Autodesk Inventor part; units mm, degrees
ref_plane "Work Plane1" through (-10, 0, -166.5) normal (-1, 0, 0) x (0, -1, 0)
ref_plane "YZ Plane" through (0, 0, 0) normal (1, 0, 0) x (0, 1, 0)
ref_plane "XZ Plane" through (0, 0, 0) normal (0, 1, 0) x (-1, 0, 0)
sketch "Sketch1" plane through (0, 0, 0) normal (1, 0, 0) x (0, 1, 0)
  line L0 (0, 0) -> (5, 0)
  line L1 (5, 0) -> (5, -15)
  line L2 (5, -15) -> (10, -15)
  line L3 (10, -15) -> (10, -72)
  line L4 (10, -72) -> (15, -72)
  line L5 (15, -72) -> (15, -121.5)
  line L6 (15, -121.5) -> (10, -121.5)
  line L7 (10, -121.5) -> (10, -166.5)
  line L8 (10, -166.5) -> (0, -166.5)
  line L9 (0, -166.5) -> (0, -166.5)
  line L10 (0, -166.5) -> (0, -166.5)
  line L11 (0, -166.5) -> (0, 0)
  point P0 (0, -83.25)
  point P1 (15, -96.75)
  point P2 (5, -166.5)
  point P3 (2.5, 0)
  point P4 (12.5, -72)
  dimension "d0" = 15
  dimension "d1" = 5
  dimension "d3" = 10
  dimension "d4" = 49.5
  dimension "d5" = 15
  dimension "d6" = 45
  dimension "d7" = 0
  dimension "d8" = 0
  dimension "d9" = 72
revolve "Revolution1" add sketch "Sketch1" angle 360 about axis through (0, 0, -166.5) along (0, 0, 1)
sketch "Sketch2" plane through (0, 0, 0) normal (0, 0, 1) x (1, 0, 0)
  circle A0 centre (0, 0) radius 5
hole "Hole1" at (0, 0, 0) direction (0, 0, -1) diameter 5.9175 depth 19.1 tip angle 118
sketch "Sketch3" plane through (0, 0, -166.5) normal (0, 0, -1) x (-1, 0, 0)
  circle A0 centre (0, 0) radius 10
  line L0 (0, 0) -> (10, 0)
  circle A1 centre (0, 0) radius 10
ref_plane "Work Plane1" through (-10, 0, -166.5) normal (-1, 0, 0) x (0, -1, 0)
sketch "Sketch4" plane through (-10, 0, -166.5) normal (-1, 0, 0) x (0, -1, 0)
  line L0 (10, 45) -> (-10, 45)
  line L1 (10, 0) -> (-10, 0)
  line L2 (10, 0) -> (-10, 0)
  line L3 (0, 0) -> (-5.5, 0)
  line L4 (-5.5, 0) -> (-5.5, 13)
  line L5 (-5.5, 13) -> (5.5, 13) construction
  line L6 (5.5, 13) -> (5.5, 0)
  line L7 (0, 0) -> (5.5, 0)
  arc A0 (5.5, 13) -> (-5.5, 13) centre (0, 13) ccw
  point P0 (0, 166.5)
  point P1 (-5.5, 0)
  dimension "d18" = 5.5
  dimension "d19" = 13
  dimension "d20" = 11
extrude "Extrusion1" cut sketch "Sketch4" against normal blind 3
sketch "Sketch5" plane through (-7, -5.5, -166.5) normal (0, 0, -1) x (-1, 0, 0)
  point P0 (-7, 5.5)
  point P1 (-7, 5.5)
hole "Hole2" at (0, 0, -166.5) direction (0, 0, 1) diameter 5.9175 depth 19.1 tip angle 118
properties part number "SP002" material "Steel, Mild"
The listing builds one solid part. Answer for the finished solid, in the listing's coordinates (mm). A direction names the side the tool comes from. Coordinates: 2 decimals unless noted, no trailing zeros. Loops run counter-clockwise (first coordinate to the right, second up) from the corner with the lowest first, then second, coordinate; pieces in that order, holes last. Notation, with made-up numbers: (61.25, 29.5) -> (106.25, 29.5) arc R15 cw to (106.25, 43.5) -> close; hole circle Ø10 at (88, -7.5). An arc over 180 degrees is marked (long way). Answer in a Markdown table with one row per item. Add a question column.
1. Flat-ended cylindrical pins translate along their axes: P1, Ø1.5, axis at y = 4, z = -50, coming from the +X side; P2, Ø2, axis at y = 9.5, z = -44, coming from the +X side; P3, Ø6, axis at y = -8, z = -128.5, coming from the -X side. Find the tip coordinate at first contact, or state that the pin passes through.
2. The part is cut by section D-D, the plane z = -79. Write down the section's boundary in (x, y).
3. The part is cut by section B-B, the plane z = -132. Write down the section's boundary in (x, y), then the cut area to 3 significant figures.
4. Determine the mould class of faces 1 (the flat face through (-5, 2, -15)), 2 (the conical face through (-0.5, 0.11, -20.57)), 3 (the cylindrical face through (9.915, -1.302, -144.315)) for opening direction Y: +Y half, -Y half, draft (parallel to the pull), parting line (faces both ways), or undercut.
5. Consider line 1 (X direction, y = 0, z = -8.25); line 2 (Y direction, x = 0, z = -157). Determine where each line is inside the solid, lowest interval first. Write a range as [from, to].
6. The part is cut by section C-C, the plane y = 11.5. Write down the section's boundary in (x, z), then the cut area to 3 significant figures.
7. The part is cut by section A-A, the plane z = -12. Write down the section's boundary in (x, y).
8. For faces 4 (the flat face through (3, 2, -166.5)), 5 (the flat face through (2.2, 2.2, 0)), 6 (the cylindrical face through (-2.934, -0.385, -156.816)), 7 (the cylindrical face through (-8, 0, -148)), 8 (the cylindrical face through (-2.934, 0.385, -9.684)), determine the directions among +Z, -Z, +X, -X, +Y, -Y from which every point of the face is accessible in a straight line to the end or side of a thin tool.
Answer below:
| question | item | result |
|---|---|---|
| 1 | P1 | x = 9.46 |
| 1 | P2 | x = 5.27 |
| 1 | P3 | x = -8.66 |
| 2 | outline | circle Ø30 at (0, 0) |
| 3 | outline | circle Ø20 at (0, 0) |
| 3 | area | 314 mm2 |
| 4 | face 1 | draft |
| 4 | face 2 | undercut |
| 4 | face 3 | parting line |
| 5 | line 1 | [-5, -2.96], [2.96, 5] |
| 5 | line 2 | [-10, -2.96], [2.96, 10] |
| 6 | outline | (-9.63, -121.5) -> (9.63, -121.5) -> (9.63, -72) -> (-9.63, -72) -> close |
| 6 | area | 953 mm2 |
| 7 | outline | circle Ø10 at (0, 0); hole circle Ø5.92 at (0, 0) |
| 8 | face 4 | -Z, +X, -X, +Y, -Y |
| 8 | face 5 | +Z, +X, -X, +Y, -Y |
| 8 | face 6 | -Z |
| 8 | face 7 | -Z, -X |
| 8 | face 8 | +Z |
